Autodesk Inventor part; units mm, degrees
ref_plane "YZ Plane" through (0, 0, 0) normal (1, 0, 0) x (0, 1, 0)
ref_plane "XZ Plane" through (0, 0, 0) normal (0, 1, 0) x (-1, 0, 0)
ref_plane "XY Plane" through (0, 0, 0) normal (0, 0, 1) x (1, 0, 0)
sketch "Sketch1" plane through (0, 0, 0) normal (0, 0, 1) x (1, 0, 0)
  circle A0 centre (0, 12.7) radius 4.0132
  circle A1 centre (-7.62, 0) radius 1.7145
  circle A2 centre (7.62, 0) radius 1.7145
  circle A3 centre (0, 0) radius 9.525
  arc A4 (-28.992, -3.5622) -> (28.992, -3.5622) centre (0, 0) ccw
  line L0 (-16.51, 12.7) -> (-16.51, 3.175)
  line L1 (16.51, 12.7) -> (16.51, 3.175)
  line L2 (19.685, 0) -> (25.8407, 0)
  line L3 (-19.685, 0) -> (-25.8407, 0)
  arc A5 (16.51, 12.7) -> (-16.51, 12.7) centre (0, 12.7) ccw
  arc A6 (-25.8407, 0) -> (-28.992, -3.5622) centre (-25.8407, -3.175) ccw
  arc A7 (-19.685, 0) -> (-16.51, 3.175) centre (-19.685, 3.175) ccw
  arc A8 (16.51, 3.175) -> (19.685, 0) centre (19.685, 3.175) ccw
  arc A9 (28.992, -3.5622) -> (25.8407, 0) centre (25.8407, -3.175) ccw
  circle A10 centre (0, 12.7) radius 9.398
  circle A11 centre (0, 0) radius 2.4765
  circle A12 centre (0, 0) radius 6.35
  line L4 (-33.494, 36.419) -> (33.7251, 36.419)
  line L5 (33.7251, 36.419) -> (33.7251, -39.9461)
  line L6 (33.7251, -39.9461) -> (-33.494, -39.9461)
  line L7 (-33.494, -39.9461) -> (-33.494, 36.419)
  circle A13 centre (0, 0) radius 10.3505
  circle A14 centre (-7.62, 0) radius 0.7937
  circle A15 centre (0, 0) radius 0.7937
  circle A16 centre (7.62, 0) radius 0.7937
  circle A17 centre (0, 12.7) radius 0.7937
  line L8 (-16.8374, 12.7) -> (-16.8374, 3.175)
  arc A18 (-19.685, 0.3274) -> (-16.8374, 3.175) centre (-19.685, 3.175) ccw
  line L9 (-19.685, 0.3274) -> (-25.8407, 0.3274)
  arc A19 (-25.8407, 0.3274) -> (-29.3169, -3.6021) centre (-25.8407, -3.175) ccw
  arc A20 (-29.3169, -3.6021) -> (29.3169, -3.6021) centre (0, 0) ccw
  arc A21 (29.3169, -3.6021) -> (25.8407, 0.3274) centre (25.8407, -3.175) ccw
  line L10 (25.8407, 0.3274) -> (19.685, 0.3274)
  arc A22 (16.8374, 3.175) -> (19.685, 0.3274) centre (19.685, 3.175) ccw
  line L11 (16.8374, 3.175) -> (16.8374, 12.7)
  arc A23 (16.8374, 12.7) -> (-16.8374, 12.7) centre (0, 12.7) ccw
  point P0 (-16.51, -24.0966)
  point P1 (16.51, -24.0966)
  point P2 (-29.21, 0)
  point P3 (29.21, 0)
  point P4 (-2.1125, 9.2878)
  point P5 (2.1125, 9.2878)
  point P6 (7.0137, 6.4446)
  point P7 (-7.0137, 6.4446)
  point P8 (-6.263, 1.0478)
  point P9 (-6.263, -1.0478)
  point P10 (6.263, -1.0478)
  point P11 (6.263, 1.0478)
  point P12 (4.5198, 4.4602)
  point P13 (-4.5198, 4.4602)
  point P14 (-7.5403, 7.0906)
  point P15 (7.5403, 7.0906)
  dimension "d20" = 8.0264
  dimension "d44" = 3.175
  dimension "d57" = 18.796
  dimension "d70" = 3.429
  dimension "d73" = 29.21
  dimension "d76" = 7.62
  dimension "d77" = 7.62
  dimension "d84" = 12.7
  dimension "d85" = 4.953
  dimension "d97" = 1.5875
  dimension "d98" = 1.5875
  dimension "d99" = 1.5875
  dimension "d100" = 1.5875
  dimension "d109" = 20.701
extrude "Extrusion22" add sketch "Sketch1" along normal blind 25.4 contours A0 A13 | A0 A13 A10 | A13 A0 A3 | A0 A3 A10 A13 | A13 A10 A3 A0 | A3 A0 | A0 A3 A10 A12 | A10 A3 A13 | A10 A12 A1 A2 A3 | A12 A10 | A10 A12 A2 A1 | A12 A1 | A1 A12 | A12 A2 | A2 A12 | A6 L3 A7 L0 A5 L1 A8 L2 A9 A4 | A11 | L4 L5 L6 L7 | A23 L11 A22 L10 A21 A20 A19 L9 A18 L8
extrude "Extrusion23" cut sketch "Sketch1" along normal blind 19.304 contours A10 A3 A13 | A10 A12 A1 A2 A3 | A10 A12 A2 A1 | A12 A1 | A1 A12 | A12 A2 | A2 A12 | A11 | A14 | A15 | A16
extrude "Extrusion24" cut sketch "Sketch1" along normal blind 11.43 contours A0 A13 | A0 A13 A10 | A13 A0 A3 | A0 A3 A10 A13 | A13 A10 A3 A0 | A3 A0 | A0 A3 A10 A12 | A10 A3 A13 | A10 A12 A1 A2 A3 | A12 A10 | A10 A12 A2 A1 | A12 A1 | A1 A12 | A12 A2 | A2 A12 | A6 L3 A7 L0 A5 L1 A8 L2 A9 A4 | A11 | A14 | A15 | A16 | A17
fillet "Fillet4" radius 1.016 1 edges at (0, -10.3505, 11.43)
fillet "Fillet5" radius 25.4 4 edges at (33.7251, -39.9461, 12.7) (-33.494, -39.9461, 12.7) (-33.494, 36.419, 12.7) (33.7251, 36.419, 12.7)
properties part number "Crank on Crankshaft_3DPrint"
Read the model definition and answer for the solid it produces. Units are mm, in the model's axes. A direction names the side the tool comes from. Coordinates: 2 decimals unless noted, no trailing zeros. Write each loop counter-clockwise with the first axis right and the second up, starting at its lowest first coordinate (ties: lowest second). Pieces come first, ordered by that corner, then holes. Notation, with made-up numbers: (-30, -22) - (5, -22) arc R17 ccw to (5, 7) - close; hole circle Ø7 at (6.5, 75). An arc over 180 degrees is marked (long way). Answer as a JSON object with one key per item and string values. Group by question number.
1. Which of the six approach directions +Z, -Z, +X, -X, +Y, -Y give full straight-line access (tool end or side, diameter ignored) to faces 4 (the cylindrical face through (-28.243, -1.1, 5.635)), 5 (the cylindrical face through (8.377, -0.238, 22.309))?
2. A cutting plane is placed at B-B (z = 21.5). Determine the outline of the cut face in (x, y).
3. A cutting plane is placed at C-C (x = 23.5). Determine the outline of the cut face in (y, z).
4. A cutting plane is placed at D-D (y = -20). Determine the outline of the cut face in (x, z), plus the area to 3 significant figures.
5. A cutting plane is placed at A-A (z = 2.5). Determine the outline of the cut face in (x, y) (3 decimals).
6. Consider L1, parallel to Y at x = 0, z = 16; L2, parallel to Y at x = 0, z = 21.5; L3, parallel to Y at x = 7.62, z = 24. Determine where each line is inside the solid, lowest interval first. Write a range as [from, to].
7. The mould has two halves that part along X. Classify faces 1 (the cylindrical face through (-8.25, 0.48, 22.31)), 2 (the flat face through (-33.494, -2, 13)), 3 (the cylindrical face through (26.09, -32.7, 12.88)): +X half, -X half, draft (parallel to the pull), parting line (faces both ways), or undercut.
8. Each of these flat-tipped pins is pushed along its axis until it touches: P1, Ø1.8, axis at x = -21.5, z = 3.5, coming from the -Y side; P2, Ø4, axis at y = 16.5, z = 11.5, coming from the +X side; P3, Ø3, axis at x = 23, z = 5.5, coming from the -Y side. Where does it stop, or does it pass through?
Worked out:
{
 "1": {"face 4": "-Z", "face 5": "+Z, -Z"},
 "2": {"outline": "(-33.49, -14.55) arc R25.4 ccw to (-8.09, -39.95) - (8.33, -39.95) arc R25.4 ccw to (33.73, -14.55) - (33.73, 11.02) arc R25.4 ccw to (8.33, 36.42) - (-8.09, 36.42) arc R25.4 ccw to (-33.49, 11.02) - close; hole circle Ø1.59 at (-7.62, 0); hole circle Ø1.59 at (0, 0); hole circle Ø1.59 at (0, 12.7); hole circle Ø1.59 at (7.62, 0)"},
 "3": {"outline": "(-34.91, 0) - (-17.35, 0) - (-17.35, 11.43) - (0, 11.43) - (0, 0) - (31.39, 0) - (31.39, 25.4) - (-34.91, 25.4) - close"},
 "4": {"outline": "(-32.9, 0) - (-21.29, 0) - (-21.29, 11.43) - (21.29, 11.43) - (21.29, 0) - (33.13, 0) - (33.13, 25.4) - (-32.9, 25.4) - close", "area": "1,190 mm²"},
 "5": {"outline": "(-33.494, -14.546) arc R25.4 ccw to (-8.094, -39.946) - (8.325, -39.946) arc R25.4 ccw to (33.725, -14.546) - (33.725, 11.019) arc R25.4 ccw to (8.325, 36.419) - (-8.094, 36.419) arc R25.4 ccw to (-33.494, 11.019) - close; hole (-28.992, -3.562) arc R29.21 ccw to (28.992, -3.562) arc R3.175 ccw to (25.841, 0) - (19.685, 0) arc R3.175 cw to (16.51, 3.175) - (16.51, 12.7) arc R16.51 ccw to (-16.51, 12.7) - (-16.51, 3.175) arc R3.175 cw to (-19.685, 0) - (-25.841, 0) arc R3.175 ccw to start"},
 "6": {"L1": "y = [-39.95, -10.35], [3.3, 11.91], [13.49, 36.42]", "L2": "y = [-39.95, -0.79], [0.79, 11.91], [13.49, 36.42]", "L3": "y = [-39.95, -0.79], [0.79, 36.42]"},
 "7": {"face 1": "undercut", "face 2": "-X half", "face 3": "+X half"},
 "8": {"P1": "stops at y = -36.65", "P2": "stops at x = 33.49", "P3": "stops at y = -36.26"}
}
